Design review of the part built by this model. Coordinates are the model's own, in mm. Face numbers are marked on the shaded views. A direction names the side the tool comes from. Give positions to 0.01 mm unless a question says otherwise; leave off trailing zeros. Loops run counter-clockwise (first coordinate to the right, second up) from the corner with the lowest first, then second, coordinate; pieces in that order, holes last. Notation, with made-up numbers: (75.5, -14) - (87.5, -14) arc R24 ccw to (87.5, 17) - close; hole circle Ø8 at (-29, -27). An arc over 180 degrees is marked (long way). Put each result on its own line as item: value. Start each with the question number.
Autodesk Inventor part; units mm, degrees
ref_plane "Arbeitsebene1" through (-1.5, 0, 0) normal (1, 0, 0) x (0, 1, 0)
ref_plane "Arbeitsebene2" through (1.5, 0, 0) normal (1, 0, 0) x (0, 1, 0)
ref_plane "Arbeitsebene3" through (-0.5, 0, 0) normal (1, 0, 0) x (0, 1, 0)
sketch "Skizze3" plane through (0, 0, 0) normal (0, 1, 0) x (-1, 0, 0)
  circle A0 centre (0, 0) radius 3
  dimension "Durchmesser" = 6
extrude "Extrusion2" add sketch "Skizze3" along normal blind 11
sketch "Skizze4" plane through (0, 0, 0) normal (0, -1, 0) x (1, 0, 0)
  circle A0 centre (0, 1.27) radius 0.5
  circle A1 centre (0, -1.27) radius 0.5
  point P0 (0, 0)
  dimension "d6" = 1
  dimension "d7" = 1
  dimension "BeinAbstand" = 2.54
  dimension "BeinZuMitte" = 1.27
extrude "Extrusion3" add sketch "Skizze4" along normal blind 4
ref_plane "Arbeitsebene1" through (-1.5, 0, 0) normal (1, 0, 0) x (0, 1, 0)
ref_plane "Arbeitsebene2" through (1.5, 0, 0) normal (1, 0, 0) x (0, 1, 0)
split_face "Trennen1"
split_face "Trennen2"
ref_plane "Arbeitsebene3" through (-0.5, 0, 0) normal (1, 0, 0) x (0, 1, 0)
ref_plane "Arbeitsebene4" through (0.5, 0, 0) normal (1, 0, 0) x (0, 1, 0)
ref_plane "Arbeitsebene5" through (0, 9, 0) normal (0, 1, 0) x (1, 0, 0)
ref_plane "Arbeitsebene6" through (0, 6.5, 0) normal (0, 1, 0) x (1, 0, 0)
sketch "Skizze5" plane through (0, 11, 0) normal (0, 1, 0) x (1, 0, 0)
  circle A0 centre (0, 0) radius 2.25
  dimension "d21" = 4.5
extrude "Extrusion4" cut sketch "Skizze5" against normal blind 0.1
split_face "Trennen3"
split_face "Trennen4"
split_face "Trennen7"
split_face "Trennen8"
ref_plane "Arbeitsebene9" through (0, 3.5, 0) normal (0, -1, 0) x (1, 0, 0)
ref_plane "Arbeitsebene10" through (0, 1, 0) normal (0, -1, 0) x (1, 0, 0)
split_face "Trennen9"
split_face "Trennen10"
sketch "Skizze6" plane through (0, 10.9, 0) normal (0, 1, 0) x (1, 0, 0)
  line L0 (1.5, -0.025) -> (0, -0.025)
  line L1 (0, -0.025) -> (0, 0.025)
  line L2 (0, 0.025) -> (1.5, 0.025)
  line L3 (1.5, 0.025) -> (1.5, -0.025)
  line L4 (0.025, 1.5) -> (0.025, 0)
  line L5 (-0.025, 0) -> (-0.025, 1.5)
  line L6 (0.025, 0) -> (-0.025, 0)
  line L7 (-0.025, 1.5) -> (0.025, 1.5)
  line L8 (-1.5, 0.025) -> (0, 0.025)
  line L9 (0, -0.025) -> (-1.5, -0.025)
  line L10 (0, 0.025) -> (0, -0.025)
  line L11 (-1.5, -0.025) -> (-1.5, 0.025)
  line L12 (-0.025, -1.5) -> (-0.025, 0)
  line L13 (0.025, 0) -> (0.025, -1.5)
  line L14 (-0.025, 0) -> (0.025, 0)
  line L15 (0.025, -1.5) -> (-0.025, -1.5)
  point P0 (0, 0)
  point P1 (0, 0)
  point P2 (0, 0)
  point P3 (0, 0)
  dimension "d26" = 0.05
  dimension "d27" = 0.025
  dimension "d28" = 1.5
  dimension "d31" = 360
extrude "Extrusion5" cut sketch "Skizze6" against normal blind 0.05
chamfer "Fase1" distance 0.05 angle 45 12 edges at (-0.025, 10.9, 0.7625) (0, 10.9, 1.5) (0.025, 10.9, 0.7625) (-0.7625, 10.9, 0.025) (-0.7625, 10.9, -0.025) (-0.025, 10.9, -0.7625) (0.025, 10.9, -0.7625) (0.7625, 10.9, 0.025) (0.7625, 10.9, -0.025) (0, 10.9, -1.5) (-1.5, 10.9, 0) (1.5, 10.9, 0)
fillet_without_effect "Rundung1"
properties part number "Kondensator"
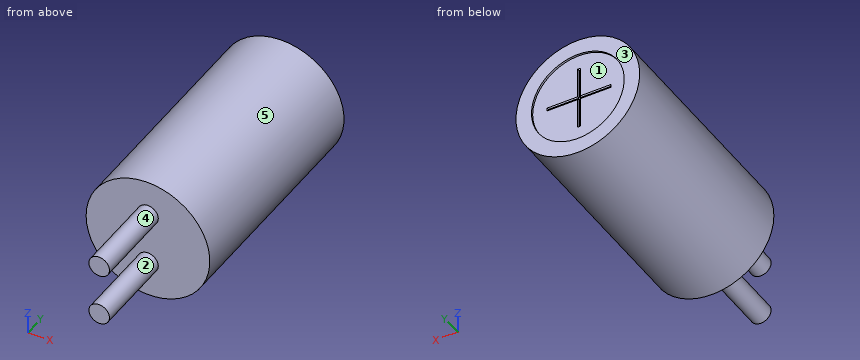
Item 1: Mouldability with a two-part tool opening along X and no side actions: class the marked faces 1, 2 and 3 as pulls with the +X half, pulls with the -X half, needs draft (parallel to the pull), parting line crosses it, or undercut.
Item 2: For L1, parallel to Y at x = -2.2, z = 1.9; L2, parallel to Z at x = -2.6, y = 3.5; L3, parallel to Y at x = 2, z = 0.1, list the stretches that pass through material, from the lowest coordinate up. Write a range as from..to.
Item 3: Consider section C-C (y = 8.25). State the section outline as (x, z) points.
Item 4: Machinability: for the marked faces 4 and 5, which of the approach directions +Z, -Z, +X, -X, +Y, -Y give a long, thin tool a straight path to every point of the face, cutting with its end or side? Answer none if there is none.
Item 5: For P1, Ø2.5, axis at x = 0.5, z = -0.5, coming from the +Y side; P2, Ø1.5, axis at y = 2, z = -1, coming from the -X side, all flat-tipped, find the tip position at first contact; note any pin that passes through.
Item 6: Consider section D-D (x = 1.75). State the section outline as (y, z) points, plus the area to 3 significant figures.
Geometry says:
1. face 1: undercut
1. face 2: parting line crosses it
1. face 3: needs draft
2. L1: y = 0..11
2. L2: z = -1.5..1.5
2. L3: y = 0..10.9
3. outline: circle Ø6 at (0, 0)
4. face 4: -Y
4. face 5: +Y, -Y
5. P1: stops at y = 10.9
5. P2: stops at x = -2.99
6. outline: (0, -2.44) - (11, -2.44) - (11, -1.41) - (10.9, -1.41) - (10.9, 1.41) - (11, 1.41) - (11, 2.44) - (0, 2.44) - close
6. area: 53.3 mm2
